For this review, take the finished solid that the model builds, in its own axes (mm). Give positions to 0.01 mm unless a question says otherwise; leave off trailing zeros. Order: outer loops, then holes, each group sorted by start corner. A loop starts at its lowest first (then second) coordinate and runs counter-clockwise, first axis right, second up.
Item 1: Consider section D-D (z = 23). Give the boundary of the cut face in (x, y).
Item 2: Consider section C-C (z = 35). Give the boundary of the cut face in (x, y).
Item 3: Consider section B-B (x = -12.5). Give the boundary of the cut face in (y, z).
Item 4: For probe 1 along X at (y, z) = (-11.5, 13.5); probe 2 along X at (y, z) = (15, 1.5); probe 3 along Z at (x, y) = (-10.5, -19.5), list the stretches that pass through material, from the lowest coordinate up.
Item 5: Consider section A-A (y = 5). Give the boundary of the cut face in (x, z), plus the area to 3 significant figures.
Item 6: For P1, Ø1, axis at x = 0, z = 25.5, coming from the +Y side; P2, Ø8, axis at y = -3.5, z = 8, coming from the -X side; P3, Ø8, axis at x = 6, y = -15, coming from the +Z side, all flat-tipped, find the tip position at first contact; note any pin that passes through.
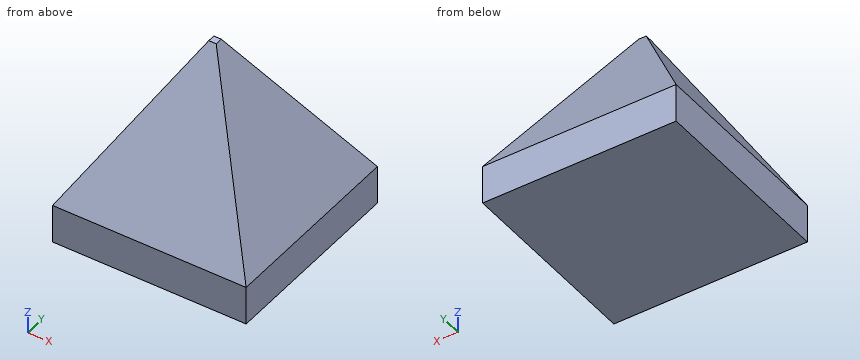
```python
from build123d import *

# Parameters (mm, degrees)
CELLULE_W          = 50
CELLULE_H          = 50
BOSS_EXTRU_1_DEPTH = 10
ESQUISSE2_W        = 50
ESQUISSE2_H        = 50
BOSS_EXTRU_2_DEPTH = 40
BOSS_EXTRU_2_TAPER = 31


with BuildPart() as part:
    # cellule → Boss.-Extru.1 (new body)
    with BuildSketch(Plane.XY):
        Rectangle(CELLULE_W, CELLULE_H)
    extrude(amount=-BOSS_EXTRU_1_DEPTH)

    # Esquisse2 → Boss.-Extru.2 (add)
    with BuildSketch(Plane.XY):
        Rectangle(ESQUISSE2_W, ESQUISSE2_H)
    extrude(amount=BOSS_EXTRU_2_DEPTH, taper=BOSS_EXTRU_2_TAPER)


solid = part.part
```
Resolved:
1. outline: (-11.18, -11.18) - (11.18, -11.18) - (11.18, 11.18) - (-11.18, 11.18) - close
2. outline: (-3.97, -3.97) - (3.97, -3.97) - (3.97, 3.97) - (-3.97, 3.97) - close
3. outline: (-25, -10) - (25, -10) - (25, 0) - (12.5, 20.8) - (-12.5, 20.8) - (-25, 0) - close
4. probe 1: x = -16.89 to 16.89
4. probe 2: x = -24.1 to 24.1
4. probe 3: z = -10 to 9.15
5. outline: (-25, -10) - (25, -10) - (25, 0) - (5, 33.29) - (-5, 33.29) - (-25, 0) - close
5. area: 1,500 mm2
6. P1: stops at y = 9.98
6. P2: stops at x = -22.6
6. P3: stops at z = 23.3
